```python
from build123d import *

# Parameters (mm, degrees)
BOSS_EXTRUDE1_DEPTH = 6.35
SKETCH4_R           = 2
SKETCH4_R_2         = 2.5
SKETCH4_R_3         = 3.175
SKETCH4_W           = 25.4
SKETCH4_H           = 6.223
CUT_EXTRUDE3_DEPTH  = 423.215315331
SKETCH5_W           = 215.9
SKETCH5_H           = 279.4
BOSS_EXTRUDE2_DEPTH = 6.35


with BuildPart() as part:
    # Sketch1 → Boss-Extrude1 (new body)
    with BuildSketch(Plane(origin=(0, 0, 0), x_dir=(1, 0, 0), z_dir=(0, 1, 0))):
        Polygon((292.1, 0), (292.1, 152.4), (228.6, 152.4), (228.6, 12.7), (12.7, 12.7), (12.7, 152.4), (0, 152.4), (0, 0), (247.65, 0), (247.65, 6.223), (273.05, 6.223), (273.05, 0), align=None)
        Polygon((228.6, 152.4), (292.1, 152.4), (292.1, 304.8), (273.05, 304.8), (273.05, 298.577), (247.65, 298.577), (247.65, 304.8), (0, 304.8), (0, 152.4), (12.7, 152.4), (12.7, 292.1), (228.6, 292.1), align=None)
    extrude(amount=BOSS_EXTRUDE1_DEPTH)

    # Sketch4 → Cut-Extrude3 (cut, through all)
    with BuildSketch(Plane(origin=(0, 6.35, 0), x_dir=(1, 0, 0), z_dir=(0, 1, 0))):
        with Locations(Location((286.6, 188.9, 0), (0, 0, 270))):
            Circle(SKETCH4_R)
        with Locations(Location((286.6, 157.9, 0), (0, 0, 270))):
            Circle(SKETCH4_R)
        with Locations(Location((255.6, 157.9, 0), (0, 0, 270))):
            Circle(SKETCH4_R)
        with Locations(Location((255.6, 188.9, 0), (0, 0, 270))):
            Circle(SKETCH4_R)
        with Locations(Location((255.6, 146.9, 0), (0, 0, 270))):
            Circle(SKETCH4_R)
        with Locations(Location((286.6, 146.9, 0), (0, 0, 270))):
            Circle(SKETCH4_R)
        with Locations(Location((284.763488048, 115.9, 0), (0, 0, 270))):
            Circle(SKETCH4_R)
        with Locations(Location((255.6, 115.9, 0), (0, 0, 270))):
            Circle(SKETCH4_R)
        with Locations(Location((271.1, 173.4, 0), (0, 0, 270))):
            Circle(SKETCH4_R_2)
        with Locations(Location((271.1, 131.4, 0), (0, 0, 270))):
            Circle(SKETCH4_R_2)
        with Locations(Location((241.3, 152.4, 0), (0, 0, 270))):
            Circle(SKETCH4_R_3)
        with Locations((260.35, 301.6885)):
            Rectangle(SKETCH4_W, SKETCH4_H)
        with Locations((260.35, 3.1115)):
            Rectangle(SKETCH4_W, SKETCH4_H)
        with Locations((31.75, 3.1115)):
            Rectangle(SKETCH4_W, SKETCH4_H)
        with Locations((31.75, 301.6885)):
            Rectangle(SKETCH4_W, SKETCH4_H)
    extrude(amount=-CUT_EXTRUDE3_DEPTH, mode=Mode.SUBTRACT)

    # Sketch5 → Boss-Extrude2 (add)
    with BuildSketch(Plane(origin=(0, 6.35, 0), x_dir=(1, 0, 0), z_dir=(0, 1, 0))):
        with Locations((120.65, 152.4)):
            Rectangle(SKETCH5_W, SKETCH5_H)
    extrude(amount=-BOSS_EXTRUDE2_DEPTH)


solid = part.part
```
For this review, take the finished solid that the model builds, in its own axes (mm). A direction names the side the tool comes from. Give positions to 0.01 mm unless a question says otherwise; leave off trailing zeros. Write each loop counter-clockwise with the first axis right and the second up, starting at its lowest first coordinate (ties: lowest second). Pieces come first, ordered by that corner, then holes.
Item 1: Wall thickness on probe 1 along X at (y, z) = (3.5, -146.9); probe 2 along X at (y, z) = (2.5, -116); probe 3 along Z at (x, y) = (255.6, 3): over which ranges is each line inside the solid? List them lowest first.
Item 2: Insertion check: P1, Ø1.9, axis at x = 29.5, y = 2.5, coming from the -Z side; P2, Ø4, axis at x = 271.1, z = -173.4, coming from the -Y side. Each pin has a flat end and moves straight along its axis. Give the tip position at first contact, or say it passes through.
Item 3: Take a section at A-A (x = 22.5). Give the boundary of the cut face in (y, z), and give its area (3 significant figures).
Item 4: The part is to be moulded in two halves that separate along X. For faces 1 (the face through (244.45, 3.22, -152.81)), 2 (the face through (144, 6.35, -155)), 3 (the face through (0, 3, -155)), say which applies: +X half, -X half, draft (parallel to the pull), parting line (faces both ways), or undercut.
Item 5: Machinability: for faces 4 (the face through (260, 3, -6.223)), 5 (the face through (261, 3, -298.577)), 6 (the face through (144, 0, -155)), which of the approach directions +Z, -Z, +X, -X, +Y, -Y give a long, thin tool a straight path to every point of the face, cutting with its end or side? Answer none if there is none.
Established:
1. probe 1: x = 0 to 253.6, 257.6 to 284.6, 288.6 to 292.1
1. probe 2: x = 0 to 253.6, 257.6 to 282.77, 286.76 to 292.1
1. probe 3: z = -298.58 to -190.9, -186.9 to -159.9, -155.9 to -148.9, -144.9 to -117.9, -113.9 to -6.22
2. P1: stops at z = -298.58
2. P2: passes through
3. outline: (0, -298.58) - (6.35, -298.58) - (6.35, -6.22) - (0, -6.22) - close
3. area: 1,860 mm2
4. face 1: undercut
4. face 2: draft
4. face 3: -X half
5. face 4: +Z, +Y, -Y
5. face 5: -Z, +Y, -Y
5. face 6: +Z, -Z, +X, -X, -Y
